```python
from build123d import *

# Parameters (mm, degrees)
SKETCH1_R           = 9.5
SKETCH1_R_2         = 6
BOSS_EXTRUDE1_DEPTH = 12
BOSS_EXTRUDE2_DEPTH = 1
CIRPATTERN1_COUNT   = 2
SKETCH3_R           = 6
SKETCH3_R_2         = 3
BOSS_EXTRUDE3_DEPTH = 2


with BuildPart() as part:
    # Sketch1 → Boss-Extrude1 (new body)
    with BuildSketch(Plane(origin=(0, 0, 0), x_dir=(1, 0, 0), z_dir=(0, 1, 0))):
        Circle(SKETCH1_R)
        Circle(SKETCH1_R_2, mode=Mode.SUBTRACT)
    extrude(amount=BOSS_EXTRUDE1_DEPTH)

    # Sketch2 → Boss-Extrude2 (add, symmetric)
    with BuildSketch(Plane.XY):
        Polygon((7.271324846, 12), (7.271324846, 0), (14.87673759, 0), (14.87673759, 7.945570702), (11.074031218, 12), align=None)
    boss_extrude2 = extrude(amount=BOSS_EXTRUDE2_DEPTH, both=True)

    # CirPattern1: Boss-Extrude2 ×2 about axis
    cirpattern1_axis = Axis((0, 0, 0), (0, 1, 0))
    for i in range(1, CIRPATTERN1_COUNT):
        add(boss_extrude2.rotate(cirpattern1_axis, i * 360 / CIRPATTERN1_COUNT))

    # Sketch3 → Boss-Extrude3 (add)
    with BuildSketch(Plane(origin=(0, 4, 0), x_dir=(1, 0, 0), z_dir=(0, 1, 0))):
        Circle(SKETCH3_R)
        Circle(SKETCH3_R_2, mode=Mode.SUBTRACT)
    extrude(amount=BOSS_EXTRUDE3_DEPTH)


solid = part.part
```
Could you check a few things on this model? Use its own coordinates, in mm. A direction names the side the tool comes from. Coordinates: 2 decimals unless noted, no trailing zeros. Write each loop counter-clockwise with the first axis right and the second up, starting at its lowest first coordinate (ties: lowest second). Pieces come first, ordered by that corner, then holes. Notation, with made-up numbers: (6, 16.25) -> (37, 16.25) arc R19 cw to (37, 34.25) -> close; hole circle Ø7 at (76.5, -5). An arc over 180 degrees is marked (long way). Return JSON: item names as keys, results as strings.
(1) We'd pull the mould along Z, two halves only. Please class faces 5 (the cylindrical face through (-3, 5, 0)), 6 (the flat face through (-3, 6, 1)), 7 (the cylindrical face through (-0.19, 5.92, 9.5)), 8 (the flat face through (-14.877, 4, 0)): +Z half, -Z half, draft (parallel to the pull), parting line (faces both ways), or undercut.
Numbers:
{"face 5": "undercut", "face 6": "undercut", "face 7": "+Z half", "face 8": "draft"}
(2) I'm going to push flat-ended pins straight in: pin 1 (3 mm diameter, centred on y = 1.5, z = -6, fed in from -X); pin 2 (6 mm diameter, centred on x = 9.5, y = 6, fed in from +Z); pin 3 (1.5 mm diameter, centred on x = -5, y = 3.5, fed in from +Z); pin 4 (5.5 mm diameter, centred on x = 0, z = 0, fed in from +Y). Where does each tip first touch, or does it pass through?
Numbers:
{"pin 1": "stops at x = -8.37", "pin 2": "stops at z = 6.93", "pin 3": "stops at z = 8.5", "pin 4": "passes through"}
(3) Imagine slicing it at D-D, the plane y = 7.5. Please give me the cut outline in (x, z), then the cut area to 3 significant figures.
Numbers:
{"outline": "(-14.88, -1) -> (-9.45, -1) arc R9.5 ccw to (9.45, -1) -> (14.88, -1) -> (14.88, 1) -> (9.45, 1) arc R9.5 ccw to (-9.45, 1) -> (-14.88, 1) -> close; hole circle Ø12 at (0, 0)", "area": "192 mm2"}
(4) Which directions (+Z, -Z, +X, -X, +Y, -Y) give clear straight access to the entire face, cutting with the end or side of a thin tool? Please do faces 1 (the flat face through (12, 6, 1)), 2 (the cylindrical face through (-6, 2, 0)), 3 (the cylindrical face through (-6, 9, 0)), 4 (the flat face through (12, 6, -1)).
Numbers:
{"face 1": "+Z, +X, +Y, -Y", "face 2": "-Y", "face 3": "+Y", "face 4": "-Z, +X, +Y, -Y"}
(5) Imagine slicing it at B-B, the plane y = 4.75. Please give me the cut outline in (x, z).
Numbers:
{"outline": "(-14.88, -1) -> (-9.45, -1) arc R9.5 ccw to (9.45, -1) -> (14.88, -1) -> (14.88, 1) -> (9.45, 1) arc R9.5 ccw to (-9.45, 1) -> (-14.88, 1) -> close; hole circle Ø6 at (0, 0)"}
(6) I need wall thicknesses on L1, parallel to Z at x = 0, y = 2; L2, parallel to X at y = 0.85, z = 0; L3, parallel to Z at x = 0, y = 5.1. Which ranges of each line are inside material? Lowest first, please.
Numbers:
{"L1": "z = -9.5 to -6, 6 to 9.5", "L2": "x = -14.88 to -6, 6 to 14.88", "L3": "z = -9.5 to -3, 3 to 9.5"}
(7) Imagine slicing it at C-C, the plane z = 0. Please give me the cut outline in (x, y), then the cut area to 3 significant figures.
Numbers:
{"outline": "(-14.88, 0) -> (-6, 0) -> (-6, 4) -> (-3, 4) -> (-3, 6) -> (-6, 6) -> (-6, 12) -> (-11.07, 12) -> (-14.88, 7.95) -> close; (3, 4) -> (6, 4) -> (6, 0) -> (14.88, 0) -> (14.88, 7.95) -> (11.07, 12) -> (6, 12) -> (6, 6) -> (3, 6) -> close", "area": "210 mm2"}
(8) Imagine slicing it at A-A, the plane x = 0. Please give me the cut outline in (y, z), then the cut area to 3 significant figures.
Numbers:
{"outline": "(0, -9.5) -> (12, -9.5) -> (12, -6) -> (6, -6) -> (6, -3) -> (4, -3) -> (4, -6) -> (0, -6) -> close; (0, 6) -> (4, 6) -> (4, 3) -> (6, 3) -> (6, 6) -> (12, 6) -> (12, 9.5) -> (0, 9.5) -> close", "area": "96.0 mm2"}
